Verification items for the finished model (mm, model axes). Face numbers are marked on the shaded views. A direction names the side the tool comes from. Give positions to 0.01 mm unless a question says otherwise; leave off trailing zeros. Write each loop counter-clockwise with the first axis right and the second up, starting at its lowest first coordinate (ties: lowest second). Pieces come first, ordered by that corner, then holes. Notation, with made-up numbers: (17.25, 47) - (28.25, 47) arc R25 ccw to (28.25, 76) - close; hole circle Ø9 at (-15.5, -10.5). An arc over 180 degrees is marked (long way). Answer as a JSON object with one key per item and string values. Group by question number.
Item 1: Sectioned sample at D-D, the plane x = 19. Record the boundary of the cut face in (y, z), and give its area (3 significant figures).
Item 2: Go/stop test with flat-tipped pins: pin 1 (10 mm diameter, centred on y = -20, z = 27, fed in from -X); pin 2 (5 mm diameter, centred on y = -18, z = -15.5, fed in from +X); pin 3 (23 mm diameter, centred on x = 0, z = 0, fed in from -Y). Record where each tip stops, or that it passes through.
Item 3: Draft check along Z on the marked faces 1, 2 and 3. Enter one of: +Z half, -Z half, draft (parallel to the pull), parting line (faces both ways), or undercut.
Item 4: Tool access check on the marked faces 4, 5 and 6. Record the directions out of +Z, -Z, +X, -X, +Y, -Y that give a thin tool (end or side, any length) a straight path to the whole face; none if there is none.
Item 5: Sectioned sample at C-C, the plane z = -28.5. Record the boundary of the cut face in (x, y).
Item 6: Sectioned sample at A-A, the plane y = -10.25. Record the boundary of the cut face in (x, z).
Item 7: Scan lines: line 1 along Y through (x, z) = (21.5, -13.5); line 2 along X through (y, z) = (-9.5, 1.5); line 3 along X through (y, z) = (-9, -8.5). Record each from-to range of solid material in increasing order. Write a range as [from, to].
Item 8: Sectioned sample at B-B, the plane x = 9. Record the boundary of the cut face in (y, z), and give its area (3 significant figures).
```python
from build123d import *

# Parameters (mm, degrees)
F0_R            = 40
F1_DEPTH        = 25
F3_DEPTH        = 25
F3_COPIES_COUNT = 8
F4_R            = 10.0757297648
F5_DEPTH        = 25
F7_DEPTH        = 5.4


# Not quite as in the source:
# - a pattern or mirror of a feature is missing from the dataset's text; its kind, count and spacing are read off the source's solid


with BuildPart() as f1:
    # F0 (on Front) → F1 (new body)
    with BuildSketch(Plane.XZ):
        Circle(F0_R)
    extrude(amount=F1_DEPTH)

    # F2 (on face) → F3 (cut)
    with BuildSketch(Plane.XZ.offset(25)):
        with BuildLine():
            ThreePointArc((0, 40), (-1.5010572917, 39.971825415), (-3, 39.8873413504))
            Line((-3, 39.8873413504), (0, 36))
            Line((0, 36), (0, 40))
        make_face()
        with BuildLine():
            Line((0, 36), (3, 39.8873413504))
            ThreePointArc((3, 39.8873413504), (1.5010572917, 39.971825415), (0, 40))
            Line((0, 40), (0, 36))
        make_face()
    f3 = extrude(amount=-F3_DEPTH, mode=Mode.SUBTRACT)

    # F3_copies: F3 ×8 about axis
    f3_copies_axis = Axis((0, 0, 0), (0, 1, 0))
    for i in range(1, F3_COPIES_COUNT):
        add(f3.rotate(f3_copies_axis, i * 360 / F3_COPIES_COUNT), mode=Mode.SUBTRACT)

    # F4 (on face) → F5 (cut)
    with BuildSketch(Plane.XZ.offset(25)):
        Circle(F4_R)
    extrude(amount=-F5_DEPTH, mode=Mode.SUBTRACT)

    # F6 (on face) → F7 (cut)
    with BuildSketch(Plane.XZ.offset(25)):
        with BuildLine():
            ThreePointArc((0, 34.0096793756), (-24.0484749125, -24.0484749125), (34.0096793756, 0))
            ThreePointArc((34.0096793756, 0), (24.0484749125, 24.0484749125), (0, 34.0096793756))
        make_face()
    extrude(amount=-F7_DEPTH, mode=Mode.SUBTRACT)


solid = f1.part
```
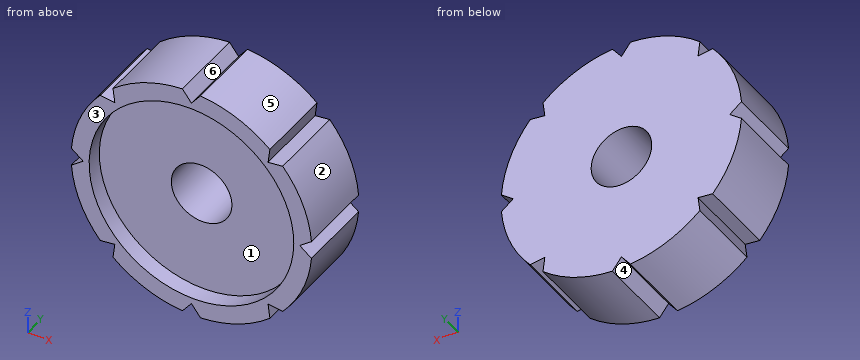
Geometry check:
{
 "1": {"outline": "(-25, -35.2) - (0, -35.2) - (0, 35.2) - (-25, 35.2) - (-25, 28.21) - (-19.6, 28.21) - (-19.6, -28.21) - (-25, -28.21) - close", "area": "1,460 mm^2"},
 "2": {"pin 1": "x = -33.41", "pin 2": "x = 37.83", "pin 3": "y = -19.6"},
 "3": {"face 1": "undercut", "face 2": "+Z half", "face 3": "draft"},
 "4": {"face 4": "-Z, +Y, -Y", "face 5": "+Z, +X, +Y, -Y", "face 6": "+Z, +Y, -Y"},
 "5": {"outline": "(-25.85, -25) - (-18.56, -25) - (-18.56, -19.6) - (18.56, -19.6) - (18.56, -25) - (25.85, -25) - (25.85, 0) - (-25.85, 0) - close"},
 "6": {"outline": "(-39.89, -3) arc R40 ccw to (-30.33, -26.08) - (-25.46, -25.46) - (-26.08, -30.33) arc R40 ccw to (-3, -39.89) - (0, -36) - (3, -39.89) arc R40 ccw to (26.08, -30.33) - (25.46, -25.46) - (30.33, -26.08) arc R40 ccw to (39.89, -3) - (36, 0) - (39.89, 3) arc R40 ccw to (30.33, 26.08) - (25.46, 25.46) - (26.08, 30.33) arc R40 ccw to (3, 39.89) - (0, 36) - (-3, 39.89) arc R40 ccw to (-26.08, 30.33) - (-25.46, 25.46) - (-30.33, 26.08) arc R40 ccw to (-39.89, 3) - (-36, 0) - close; hole circle Ø20.15 at (0, 0)"},
 "7": {"line 1": "[-19.6, 0]", "line 2": "[-37.94, -9.96], [9.96, 37.94]", "line 3": "[-39.09, -5.41], [5.41, 39.09]"},
 "8": {"outline": "(-25, -38.97) - (0, -38.97) - (0, -4.53) - (-19.6, -4.53) - (-19.6, -32.8) - (-25, -32.8) - close; (-25, 32.8) - (-19.6, 32.8) - (-19.6, 4.53) - (0, 4.53) - (0, 38.97) - (-25, 38.97) - close", "area": "1,420 mm^2"}
}
